Could you check a few things on this model? Use its own coordinates, in mm. Coordinates: 2 decimals unless noted, no trailing zeros. Loops run counter-clockwise (first coordinate to the right, second up) from the corner with the lowest first, then second, coordinate; pieces in that order, holes last.
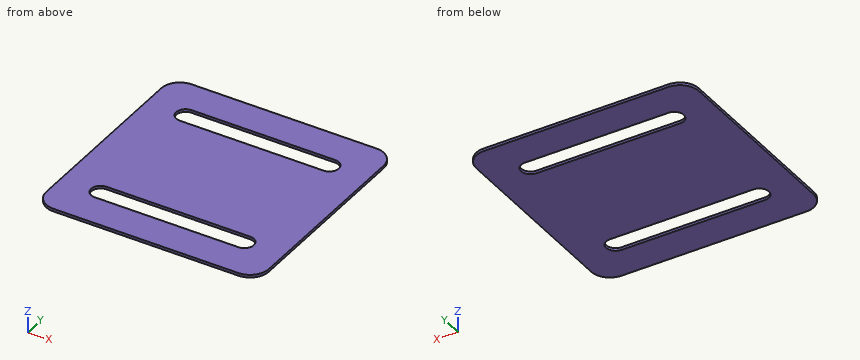
Autodesk Fusion 360 part; units mm, degrees
sketch "Sketch1" plane through (0, 0, 0) normal (0, 0, 1) x (1, 0, 0)
  line L0 (-32.5, 32.5) -> (32.5, 32.5)
  line L1 (32.5, 32.5) -> (32.5, -32.5)
  line L2 (32.5, -32.5) -> (-32.5, -32.5)
  line L3 (-32.5, -32.5) -> (-32.5, 32.5)
  line L4 (-32.5, 32.5) -> (32.5, -32.5) construction
  line L5 (32.5, 32.5) -> (-32.5, -32.5) construction
  line L6 (-32.5, 0) -> (-32.5, 20) construction
  line L7 (-32.5, 20) -> (32.5, 20) construction
  line L8 (-32.5, 0) -> (-32.5, -20) construction
  line L9 (-32.5, -20) -> (32.5, -20) construction
  line L10 (-21, -22.75) -> (21, -22.75)
  arc A0 (21, -22.75) -> (21, -17.25) centre (21, -20) ccw
  line L11 (21, -17.25) -> (-21, -17.25)
  arc A1 (-21, -17.25) -> (-21, -22.75) centre (-21, -20) ccw
  line L12 (-21, -20) -> (21, -20) construction
  line L13 (-32.5, 0) -> (32.5, 0) construction
  line L14 (21, 17.25) -> (-21, 17.25)
  arc A2 (-21, 22.75) -> (-21, 17.25) centre (-21, 20) ccw
  line L15 (-21, 22.75) -> (21, 22.75)
  arc A3 (21, 17.25) -> (21, 22.75) centre (21, 20) ccw
  point P0 (0, -20)
  dimension "d1" = 65
  dimension "d2" = 65
  dimension "d3" = 5.5
extrude "Extrude1" add sketch "Sketch1" along normal blind 0.8
fillet "Fillet1" radius 5.5 4 edges at (32.5, -32.5, 0.4) (32.5, 32.5, 0.4) (-32.5, 32.5, 0.4) (-32.5, -32.5, 0.4)
1) Imagine slicing it at B-B on x = -3. List the corners of the cut face in (y, z) for me.
2) Imagine slicing it at A-A on y = -20. List the corners of the cut face in (x, z) for me, plus the area to 3 significant figures.
3) Imagine slicing it at C-C on z = 0.45. List the corners of the cut face in (x, y) for me, plus the area to 3 significant figures.
4) If I drill on L1, parallel to Y at x = 17, z = 0.65; L2, parallel to Y at x = 30, z = 0.15; L3, parallel to X at y = 21, z = 0.3, over which ranges is the centre line in solid material (lowest first)?
Solved:
1. outline: (-32.5, 0) - (-22.75, 0) - (-22.75, 0.8) - (-32.5, 0.8) - close; (-17.25, 0) - (17.25, 0) - (17.25, 0.8) - (-17.25, 0.8) - close; (22.75, 0) - (32.5, 0) - (32.5, 0.8) - (22.75, 0.8) - close
2. outline: (-32.5, 0) - (-23.75, 0) - (-23.75, 0.8) - (-32.5, 0.8) - close; (23.75, 0) - (32.5, 0) - (32.5, 0.8) - (23.75, 0.8) - close
2. area: 14.0 mm2
3. outline: (-32.5, -27) arc R5.5 ccw to (-27, -32.5) - (27, -32.5) arc R5.5 ccw to (32.5, -27) - (32.5, 27) arc R5.5 ccw to (27, 32.5) - (-27, 32.5) arc R5.5 ccw to (-32.5, 27) - close; hole (-21, -22.75) - (21, -22.75) arc R2.75 ccw to (21, -17.25) - (-21, -17.25) arc R2.75 ccw to start; hole (-21, 17.25) - (21, 17.25) arc R2.75 ccw to (21, 22.75) - (-21, 22.75) arc R2.75 ccw to start
3. area: 3,690 mm2
4. L1: y = -32.5 to -22.75, -17.25 to 17.25, 22.75 to 32.5
4. L2: y = -31.61 to 31.61
4. L3: x = -32.5 to -23.56, 23.56 to 32.5
